```python
from build123d import *

# Parameters (mm, degrees)
SKETCH_W            = 120
SKETCH_H            = 120
PAD_DEPTH           = 9
HOLE002_D           = 47.5
HOLE002_DEPTH       = 25
HOLE002_CBORE_D     = 53
HOLE002_CBORE_DEPTH = 2
CYLINDER_R          = 3.5
CYLINDER_DEPTH      = 39
HOLE003_D           = 3.23
HOLE003_CBORE_D     = 7
HOLE003_CBORE_DEPTH = 2.91


with BuildPart() as part:
    # Sketch → Pad (new body)
    with BuildSketch(Plane(origin=(0, 0, 0), x_dir=(-1, 0, 0), z_dir=(0, 0, -1))):
        with Locations((0, 60)):
            Rectangle(SKETCH_W, SKETCH_H)
    extrude(amount=PAD_DEPTH)

    # Hole002
    with Locations(Plane(origin=(0, 60, 0), x_dir=(1, 0, 0), z_dir=(0, 0, 1))):
        with Locations((0, 0)):
            CounterBoreHole(HOLE002_D / 2, HOLE002_CBORE_D / 2, HOLE002_CBORE_DEPTH, depth=HOLE002_DEPTH)

    # Cylinder → Cylinder (join)
    with BuildSketch(Plane(origin=(17, 77, 39), x_dir=(0, 1, 0), z_dir=(0, 0, 1))):
        Circle(CYLINDER_R)
    extrude(amount=CYLINDER_DEPTH)

    # Hole003 (through all)
    with Locations(Plane(origin=(0, 60, 0), x_dir=(1, 0, 0), z_dir=(0, 0, 1))):
        with Locations((17, 17)):
            CounterBoreHole(HOLE003_D / 2, HOLE003_CBORE_D / 2, HOLE003_CBORE_DEPTH)


solid = part.part
```
The model under review builds one solid part; all positions refer to its coordinate system, in mm. A direction names the side the tool comes from. Give positions to 0.01 mm unless a question says otherwise; leave off trailing zeros. Loops run counter-clockwise (first coordinate to the right, second up) from the corner with the lowest first, then second, coordinate; pieces in that order, holes last. Notation, with made-up numbers: (86, 22.25) - (124, 22.25) arc R29 cw to (124, 57.25) - close; hole circle Ø4 at (57.5, -25.5). An arc over 180 degrees is marked (long way). Answer as a JSON object with one key per item and string values.
Q1. Mouldability with a two-part tool opening along Y and no side actions: class faces 3 (the flat face through (1, 120, -4)), 4 (the cylindrical face through (18.113, 78.17, -5.998)), 5 (the flat face through (28, 61, 0)) as +Y half, -Y half, draft (parallel to the pull), parting line (faces both ways), or undercut.
Worked out:
{"face 3": "+Y half", "face 4": "undercut", "face 5": "draft"}
Q2. Insertion check: pin 1 (4 mm diameter, centred on x = 17, y = 77, fed in from +Z). The pin has a flat end and moves straight along its axis. Give the tip position at first contact, or say it passes through.
Worked out:
{"pin 1": "stops at z = -2.91"}
Q3. Add section B-B on x = 0. State the section outline as (y, z) points.
Worked out:
{"outline": "(0, -9) - (36.25, -9) - (36.25, -2) - (33.5, -2) - (33.5, 0) - (0, 0) - close; (83.75, -9) - (120, -9) - (120, 0) - (86.5, 0) - (86.5, -2) - (83.75, -2) - close"}
Q4. For faces 1 (the cylindrical face through (19.534, 79.414, -1.758)), 2 (the flat face through (-60, 59, -4)), list the 3-axis set-ups (+Z, -Z, +X, -X, +Y, -Y) from which the entire face can be reached by the end or side of a thin tool; tool diameter is ignored.
Worked out:
{"face 1": "+Z", "face 2": "+Z, -Z, -X, +Y, -Y"}
Q5. To check wall thickness, follow line 1 along X through (y, z) = (61, -4.25); line 2 along X through (y, z) = (60, -1.35); line 3 along Y through (x, z) = (0, -3.25). State the ranges of each line that lie inside material, in increasing order.
Worked out:
{"line 1": "x = -60 to -23.73, 23.73 to 60", "line 2": "x = -60 to -26.5, 26.5 to 60", "line 3": "y = 0 to 36.25, 83.75 to 120"}
Q6. Add section C-C on z = -6.25. State the section outline as (x, y) points (3 decimals), plus the area to 3 significant figures.
Worked out:
{"outline": "(-60, 0) - (60, 0) - (60, 120) - (-60, 120) - close; hole (15.641, 77.872) arc R23.75 ccw (long way) to (17.872, 75.641) arc R1.615 ccw (long way) to start", "area": "12,600 mm^2"}
Q7. Add section A-A on y = 60. State the section outline as (x, z) points.
Worked out:
{"outline": "(-60, -9) - (-23.75, -9) - (-23.75, -2) - (-26.5, -2) - (-26.5, 0) - (-60, 0) - close; (23.75, -9) - (60, -9) - (60, 0) - (26.5, 0) - (26.5, -2) - (23.75, -2) - close"}
